```python
from build123d import *

# Parameters (mm, degrees)
SKETCH1_R         = 139.7
SKETCH1_R_2       = 84.1375
EXTRUDE1_DEPTH    = 12.7
CIRPATTERN2_COUNT = 8
EXTRUDE4_DEPTH    = 98.345625
SKETCH8_R         = 6.35
EXTRUDE5_DEPTH    = 4.7625
CIRPATTERN4_COUNT = 8


with BuildPart() as part:
    # Sketch1 → Extrude1 (new body)
    with BuildSketch(Plane.XY):
        Circle(SKETCH1_R)
        Circle(SKETCH1_R_2, mode=Mode.SUBTRACT)
    extrude(amount=EXTRUDE1_DEPTH)

    # Sketch2 → 0.625_ Diameter Hole1 (revolve, cut)
    with BuildSketch(Plane(origin=(0, 120.65, 12.7), x_dir=(0, -1, 0), z_dir=(1, 0, 0))):
        Polygon((0, 0), (0, 32.077063629), (11.1125, 25.4), (11.1125, 0), align=None)
    f_0_625_diameter_hole1 = revolve(axis=Axis((0, 120.65, 19.05), (0, 0, -1)), mode=Mode.SUBTRACT)

    # CirPattern2: 0.625_ Diameter Hole1 ×8 about axis
    cirpattern2_axis = Axis((0, 0, 0), (0, 0, 1))
    for i in range(1, CIRPATTERN2_COUNT):
        add(f_0_625_diameter_hole1.rotate(cirpattern2_axis, i * 360 / CIRPATTERN2_COUNT), mode=Mode.SUBTRACT)

    # Sketch6 → Extrude4 (add)
    with BuildSketch(Plane.XY.offset(12.7)):
        Polygon((-55.596678696, 127.999749611), (-34.313207501, 76.616904797), (-29.913231227, 78.439434644), (-51.196702422, 129.822279457), align=None)
    extrude4 = extrude(amount=EXTRUDE4_DEPTH)

    # Sketch8 → Extrude5 (cut)
    with BuildSketch(Plane(origin=(2.199988137, 0.911264923, 0), x_dir=(0, 0, -1), z_dir=(0.923879533, 0.382683432, 0))):
        with Locations((-34.755447715, 105.971333923)):
            Circle(SKETCH8_R)
        Polygon((-12.7, 139.532276663), (-111.045625, 83.915886208), (-111.045625, 139.532276663), align=None)
        with BuildLine():
            Line((-12.7, 90.265886208), (-12.7, 83.915886208))
            Line((-12.7, 83.915886208), (-19.05, 83.915886208))
            ThreePointArc((-19.05, 83.915886208), (-17.190128061, 88.406014269), (-12.7, 90.265886208))
        make_face()
    extrude5 = extrude(amount=-EXTRUDE5_DEPTH, mode=Mode.SUBTRACT)

    # CirPattern4: Extrude4, Extrude5 ×8 about axis
    cirpattern4_axis = Axis((0, 0, 0), (0, 0, 1))
    for i in range(1, CIRPATTERN4_COUNT):
        add(extrude4.rotate(cirpattern4_axis, i * 360 / CIRPATTERN4_COUNT))
        add(extrude5.rotate(cirpattern4_axis, i * 360 / CIRPATTERN4_COUNT), mode=Mode.SUBTRACT)


solid = part.part
```
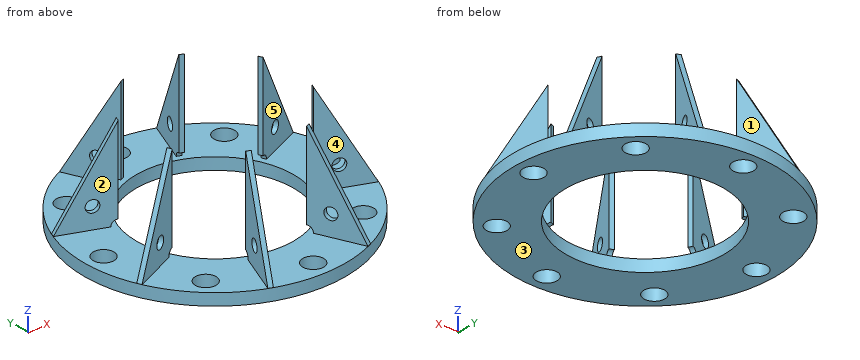
Input: part model. Units: mm. Frame: model coordinates. Face numbers are marked on the shaded views. A direction names the side the tool comes from. Coordinates: 2 decimals unless noted, no trailing zeros. Loops run counter-clockwise (first coordinate to the right, second up) from the corner with the lowest first, then second, coordinate; pieces in that order, holes last. Notation, with made-up numbers: (2, -16) -> (10, -16) arc R31 cw to (10, 8) -> close; hole circle Ø6 at (60, -14). An arc over 180 degrees is marked (long way). Use a Markdown table: item, result.
1) Material intervals for line 1 along Y through (x, z) = (0, 3); line 2 along Z through (x, y) = (-99, -67); line 3 along Y through (x, z) = (44, 48), sorted ascending. Write a range as from..to.
Results found:
| item | result |
|---|---|
| line 1 | y = -139.7..-131.76, -109.54..-84.14, 84.14..109.54, 131.76..139.7 |
| line 2 | z = 0..12.7 |
| line 3 | y = -111.2..-100, 100..111.2 |
2) Access query for the marked faces 1, 2, 3, 4 and 5. Directions: +Z, -Z, +X, -X, +Y, -Y. A direction counts if a zero-diameter tool reaches every point of the face in a straight line with its end or side. Return the directions, or none.
Results found:
| item | result |
|---|---|
| face 1 | +Z, +Y |
| face 2 | +Z, -X |
| face 3 | -Z, +X, -X, +Y, -Y |
| face 4 | +Z, -Y |
| face 5 | +Z, +X |
3) Cut plane D-D (x = -120.65). Return the cut outline in (y, z), then the cut area to 3 significant figures.
Results found:
| item | result |
|---|---|
| outline | (-70.42, 0) -> (-11.11, 0) -> (-11.11, 12.7) -> (-47.4, 12.7) -> (-47.4, 30.26) -> (-52.55, 26.77) -> (-52.55, 12.7) -> (-70.42, 12.7) -> close; (11.11, 0) -> (70.42, 0) -> (70.42, 12.7) -> (52.55, 12.7) -> (52.55, 26.77) -> (47.4, 30.26) -> (47.4, 12.7) -> (11.11, 12.7) -> close |
| area | 1,670 mm2 |
4) Cut plane C-C (z = 100.5). Give the number of separate pieces and of enclosed holes in the cut face, then the cut area to 3 significant figures.
Results found:
| item | result |
|---|---|
| separate pieces | 8 |
| enclosed holes | 0 |
| area | 227 mm2 |
5) Cut plane B-B (y = -20.5). Return the cut outline in (x, z), then the cut area to 3 significant figures.
Results found:
| item | result |
|---|---|
| outline | (-138.19, 0) -> (-81.6, 0) -> (-81.6, 12.7) -> (-138.19, 12.7) -> close; (81.6, 0) -> (138.19, 0) -> (138.19, 12.7) -> (81.6, 12.7) -> close |
| area | 1,440 mm2 |
6) Cut plane A-A (x = 0). Return the cut outline in (y, z), then the cut area to 3 significant figures.
Results found:
| item | result |
|---|---|
| outline | (-139.7, 0) -> (-131.76, 0) -> (-131.76, 12.7) -> (-139.7, 12.7) -> close; (-109.54, 0) -> (-84.14, 0) -> (-84.14, 12.7) -> (-109.54, 12.7) -> close; (84.14, 0) -> (109.54, 0) -> (109.54, 12.7) -> (84.14, 12.7) -> close; (131.76, 0) -> (139.7, 0) -> (139.7, 12.7) -> (131.76, 12.7) -> close |
| area | 847 mm2 |
7) Contact query for flat-ended pins moving along their axis: pin 1 (2 mm diameter, centred on x = 6.5, z = 12.5, fed in from -Y); pin 2 (13.5 mm diameter, centred on x = 0, y = -120.65, fed in from +Z); pin 3 (10 mm diameter, centred on x = -49.5, z = 37.5, fed in from +Y); pin 4 (4 mm diameter, centred on x = -100, z = 40.5, fed in from +Y). Output: stop coordinate, or through.
Results found:
| item | result |
|---|---|
| pin 1 | stops at y = -139.59 |
| pin 2 | passes through |
| pin 3 | stops at y = 119.04 |
| pin 4 | stops at y = 44.83 |
